Design review of the part built by this model. Coordinates are the model's own, in mm. A direction names the side the tool comes from. Coordinates: 2 decimals unless noted, no trailing zeros. Write each loop counter-clockwise with the first axis right and the second up, starting at its lowest first coordinate (ties: lowest second). Pieces come first, ordered by that corner, then holes.
Q1. To check wall thickness, follow probe 1 along X at (y, z) = (74, 29); probe 2 along Y at (x, z) = (-6.5, 56); probe 3 along Y at (x, z) = (35.5, 41). State the ranges of each line that lie inside material, in increasing order.
Q2. Add section C-C, the plane y = 267.5. Give the boundary of the cut face in (x, z), plus the area to 3 significant figures.
Q3. The part is to be moulded in two halves that separate along Y. For faces 1 (the face through (323.85, 180, 41)), 2 (the face through (-7.26, -330.12, 40.7)), 3 (the face through (-75, -316, 0)), say which applies: +Y half, -Y half, draft (parallel to the pull), parting line (faces both ways), or undercut.
Q4. Add section A-A, the plane z = 69.5. Give the boundary of the cut face in (x, y).
Q5. Add section B-B, the plane x = 0. Give the boundary of the cut face in (y, z), plus the area to 3 significant figures.
Q6. Machinability: for faces 4 (the face through (5, 361.95, 41)), 5 (the face through (-5, 355.6, 41)), which of the approach directions +Z, -Z, +X, -X, +Y, -Y give a long, thin tool a straight path to every point of the face, cutting with its end or side? Answer none if there is none.
Q7. Clearance check with flat-ended pins moving along their axes: pin 1 Ø10 at (x, z) = (156.5, 74) entering from -Y; pin 2 Ø6 at (x, z) = (236, 45) entering from -Y; pin 3 Ø5 at (y, z) = (-256.5, 36.5) entering from +X. State where each tip first meets the part, or that it passes through.
from build123d import *

# Parameters (mm, degrees)
F1_DEPTH = 82.55


with BuildPart() as f1:
    # F0 (on Top) → F1 (new body)
    with BuildSketch(Plane.XY):
        with BuildLine():
            ThreePointArc((-330.2, 0), (0, -330.2), (330.2, 0))
            Line((330.2, 0), (330.2, 361.95))
            Line((330.2, 361.95), (-330.2, 361.95))
            Line((-330.2, 361.95), (-330.2, 0))
        make_face()
        with BuildLine():
            ThreePointArc((323.85, 0), (0, -323.85), (-323.85, 0))
            Line((-323.85, 0), (-323.85, 355.6))
            Line((-323.85, 355.6), (323.85, 355.6))
            Line((323.85, 355.6), (323.85, 0))
        make_face(mode=Mode.SUBTRACT)
    extrude(amount=F1_DEPTH)


solid = f1.part
Here are the results:
1. probe 1: x = -330.2 to -323.85, 323.85 to 330.2
1. probe 2: y = -330.14 to -323.78, 355.6 to 361.95
1. probe 3: y = -328.29 to -321.9, 355.6 to 361.95
2. outline: (-330.2, 0) - (-323.85, 0) - (-323.85, 82.55) - (-330.2, 82.55) - close; (323.85, 0) - (330.2, 0) - (330.2, 82.55) - (323.85, 82.55) - close
2. area: 1,050 mm2
3. face 1: undercut
3. face 2: -Y half
3. face 3: draft
4. outline: (-330.2, 0) arc R330.2 ccw to (330.2, 0) - (330.2, 361.95) - (-330.2, 361.95) - close; hole (-323.85, 0) arc R323.85 ccw to (323.85, 0) - (323.85, 355.6) - (-323.85, 355.6) - close
5. outline: (-330.2, 0) - (-323.85, 0) - (-323.85, 82.55) - (-330.2, 82.55) - close; (355.6, 0) - (361.95, 0) - (361.95, 82.55) - (355.6, 82.55) - close
5. area: 1,050 mm2
6. face 4: +Z, -Z, +X, -X, +Y
6. face 5: +Z, -Z
7. pin 1: stops at y = -293.39
7. pin 2: stops at y = -233.97
7. pin 3: stops at x = 210.99
